Model file for the job. Use its own axes, mm. A direction names the side the tool comes from. Give positions to 0.01 mm unless a question says otherwise; leave off trailing zeros. Loops run counter-clockwise (first coordinate to the right, second up) from the corner with the lowest first, then second, coordinate; pieces in that order, holes last. Notation, with made-up numbers: (-6.75, 66) - (34.25, 66) arc R28 cw to (34.25, 89) - close; hole circle Ø3 at (66, -32.75). An arc over 180 degrees is marked (long way). Use a Markdown table: item, result.
from build123d import *

# Parameters (mm, degrees)
SKETCH1_W           = 100
SKETCH1_H           = 100
BOSS_EXTRUDE1_DEPTH = 20
CUT_EXTRUDE1_DEPTH  = 20
SKETCH6_W           = 60
SKETCH6_H           = 90
CUT_EXTRUDE2_DEPTH  = 15
SKETCH2_W           = 5
SKETCH2_H           = 100
BOSS_EXTRUDE2_DEPTH = 10
CHAMFER1_SIZE       = 10
SKETCH7_R           = 3
CUT_EXTRUDE3_DEPTH  = 50
CUT_EXTRUDE4_START  = -10
SKETCH9_R           = 7
CUT_EXTRUDE4_DEPTH  = 50
LPATTERN1_COUNT     = 2
LPATTERN1_PITCH     = 40


with BuildPart() as part:
    # Sketch1 → Boss-Extrude1 (new body)
    with BuildSketch(Plane.XY):
        with Locations((-7.788018433, -1.33640553)):
            Rectangle(SKETCH1_W, SKETCH1_H)
    extrude(amount=BOSS_EXTRUDE1_DEPTH)

    # Sketch5 → Cut-Extrude1 (cut)
    with BuildSketch(Plane.XY.offset(20)):
        with BuildLine():
            Line((31.754288081, -11.717886794), (21.754288081, -11.717886794))
            ThreePointArc((21.754288081, -11.717886794), (19.254288081, -9.217886794), (21.754288081, -6.717886794))
            Line((21.754288081, -6.717886794), (31.754288081, -6.717886794))
            ThreePointArc((31.754288081, -6.717886794), (34.254288081, -9.217886794), (31.754288081, -11.717886794))
        make_face()
        with BuildLine():
            Line((8.254288081, -5.217886794), (-1.745711919, -5.217886794))
            ThreePointArc((-1.745711919, -5.217886794), (-21.245711919, 14.282113206), (-1.745711919, 33.782113206))
            Line((-1.745711919, 33.782113206), (8.254288081, 33.782113206))
            ThreePointArc((8.254288081, 33.782113206), (27.754288081, 14.282113206), (8.254288081, -5.217886794))
        make_face()
        with BuildLine():
            Line((31.754288081, 35.035010382), (21.754288081, 35.035010382))
            ThreePointArc((21.754288081, 35.035010382), (19.007185257, 37.782113206), (21.754288081, 40.52921603))
            Line((21.754288081, 40.52921603), (31.754288081, 40.52921603))
            ThreePointArc((31.754288081, 40.52921603), (34.501390905, 37.782113206), (31.754288081, 35.035010382))
        make_face()
        with BuildLine():
            Line((-15.245711919, 35.035010382), (-25.245711919, 35.035010382))
            ThreePointArc((-25.245711919, 35.035010382), (-27.992814743, 37.782113206), (-25.245711919, 40.52921603))
            Line((-25.245711919, 40.52921603), (-15.245711919, 40.52921603))
            ThreePointArc((-15.245711919, 40.52921603), (-12.498609095, 37.782113206), (-15.245711919, 35.035010382))
        make_face()
        with BuildLine():
            Line((-15.245711919, -11.964989618), (-25.245711919, -11.964989618))
            ThreePointArc((-25.245711919, -11.964989618), (-27.992814743, -9.217886794), (-25.245711919, -6.47078397))
            Line((-25.245711919, -6.47078397), (-15.245711919, -6.47078397))
            ThreePointArc((-15.245711919, -6.47078397), (-12.498609095, -9.217886794), (-15.245711919, -11.964989618))
        make_face()
    extrude(amount=-CUT_EXTRUDE1_DEPTH, mode=Mode.SUBTRACT)

    # Sketch6 → Cut-Extrude2 (cut)
    with BuildSketch(Plane(origin=(0, 0, 0), x_dir=(-1, 0, 0), z_dir=(0, 0, -1))):
        with Locations((-7.211981567, -1.33640553)):
            Rectangle(SKETCH6_W, SKETCH6_H)
    extrude(amount=-CUT_EXTRUDE2_DEPTH, mode=Mode.SUBTRACT)

    # Sketch2 → Boss-Extrude2 (add)
    with BuildSketch(Plane(origin=(0, 0, 0), x_dir=(-1, 0, 0), z_dir=(0, 0, -1))):
        with Locations((35.288018433, -1.33640553)):
            Rectangle(SKETCH2_W, SKETCH2_H)
    extrude(amount=BOSS_EXTRUDE2_DEPTH)

    # Chamfer1
    chamfer1_edges = [part.edges().sort_by_distance(p)[0] for p in [
        (-57.788018433, -1.33640553, 20),
    ]]
    chamfer(chamfer1_edges, length=CHAMFER1_SIZE)

    # Sketch7 → Cut-Extrude3 (cut)
    with BuildSketch(Plane(origin=(0, 0, 0), x_dir=(-1, 0, 0), z_dir=(0, 0, -1))):
        with Locations((47.788018433, -41.33640553)):
            Circle(SKETCH7_R)
    cut_extrude3 = extrude(amount=-CUT_EXTRUDE3_DEPTH, mode=Mode.SUBTRACT)

    # Sketch9 → Cut-Extrude4 (cut)
    with BuildSketch(Plane(origin=(0, 0, 0), x_dir=(-1, 0, 0), z_dir=(0, 0, -1)).offset(CUT_EXTRUDE4_START)):
        with Locations((47.788018433, -41.33640553)):
            Circle(SKETCH9_R)
    cut_extrude4 = extrude(amount=-CUT_EXTRUDE4_DEPTH, mode=Mode.SUBTRACT)

    # LPattern1: Cut-Extrude3, Cut-Extrude4 ×2
    with Locations(*[(0, i * LPATTERN1_PITCH, 0) for i in range(1, LPATTERN1_COUNT)]):
        add(cut_extrude3, mode=Mode.SUBTRACT)
        add(cut_extrude4, mode=Mode.SUBTRACT)


solid = part.part
(1) Pin check, flat tips, straight feed: P1, Ø18, axis at x = -47.79, y = -1.34, coming from the -Z side; P2, Ø3.5, axis at x = -47.79, y = -41.34, coming from the +Z side; P3, Ø5, axis at y = -5, z = 16, coming from the -X side. Stop position of each tip, or through.
Computed:
| item | result |
|---|---|
| P1 | z = 0 |
| P2 | through |
| P3 | x = -54.29 |
(2) Slice it at A-A, the plane x = -24. Write the cut outline in (y, z), plus the area to 3 significant figures.
Computed:
| item | result |
|---|---|
| outline | (-51.34, 0) - (-11.96, 0) - (-11.96, 20) - (-51.34, 20) - close; (-6.47, 0) - (35.04, 0) - (35.04, 20) - (-6.47, 20) - close; (40.53, 0) - (48.66, 0) - (48.66, 20) - (40.53, 20) - close |
| area | 1,780 mm² |
(3) Slice it at D-D, the plane z = 3.5. Write the cut outline in (x, y).
Computed:
| item | result |
|---|---|
| outline | (-57.79, -51.34) - (42.21, -51.34) - (42.21, 48.66) - (-57.79, 48.66) - close; hole circle Ø6 at (-47.79, -41.34); hole circle Ø6 at (-47.79, -1.34); hole (-25.25, -11.96) - (-22.79, -11.96) - (-22.79, -46.34) - (37.21, -46.34) - (37.21, 43.66) - (-22.79, 43.66) - (-22.79, 40.53) - (-25.25, 40.53) arc R2.75 ccw to (-25.25, 35.04) - (-22.79, 35.04) - (-22.79, -6.47) - (-25.25, -6.47) arc R2.75 ccw to start |
(4) Mould opens along X. For faces 1 (the flat face through (-32.788, -2, -5)), 2 (the cylindrical face through (-40.795, -1.029, 13.819)), 3 (the flat face through (-23, -1, 0)) say: pulls with the +X half, pulls with the -X half, needs draft (parallel to the pull), parting line crosses it, or undercut.
Computed:
| item | result |
|---|---|
| face 1 | pulls with the +X half |
| face 2 | undercut |
| face 3 | needs draft |
(5) Slice it at B-B, the plane y = -17. Write the cut outline in (x, z).
Computed:
| item | result |
|---|---|
| outline | (-57.79, 0) - (-37.79, 0) - (-37.79, -10) - (-32.79, -10) - (-32.79, 0) - (-22.79, 0) - (-22.79, 15) - (37.21, 15) - (37.21, 0) - (42.21, 0) - (42.21, 20) - (-47.79, 20) - (-57.79, 10) - close |
(6) Slice it at C-C, the plane x = -10. Write the cut outline in (y, z).
Computed:
| item | result |
|---|---|
| outline | (-51.34, 0) - (-46.34, 0) - (-46.34, 15) - (-3.38, 15) - (-3.38, 20) - (-51.34, 20) - close; (31.95, 15) - (43.66, 15) - (43.66, 0) - (48.66, 0) - (48.66, 20) - (31.95, 20) - close |
(7) Drill centre lines: probe 1 along X at (y, z) = (31, 5.5); probe 2 along Y at (x, z) = (4, 14.5); probe 3 along X at (y, z) = (0.5, 4). Where is each one in solid material? Low to high. Write a range as [from, to].
Computed:
| item | result |
|---|---|
| probe 1 | [-57.79, -22.79], [37.21, 42.21] |
| probe 2 | [-51.34, -46.34], [43.66, 48.66] |
| probe 3 | [-57.79, -50.16], [-45.42, -22.79], [37.21, 42.21] |
(8) 3-axis set-ups, long thin cutter, end or side, ignore diameter. For faces 4 (the flat face through (-51, -41, 10)), 5 (the cylindrical face through (-12.5, -9.2, 17.5)), 6 (the flat face through (-52, -1, 0)): which of +Z, -Z, +X, -X, +Y, -Y reach the whole face in a straight line?
Computed:
| item | result |
|---|---|
| face 4 | +Z |
| face 5 | +Z, -Z |
| face 6 | -Z, -X, +Y, -Y |
